from build123d import *

# Parameters (mm, degrees)
EXTRUDE_1_DEPTH = 3


with BuildPart() as part:
    # 草图1 → 凸台-拉伸1 (new body)
    with BuildSketch(Plane.XY):
        Polygon((120, -3), (80, -3), (80, 0), (61.5, 0), (61.5, -3), (62.75, -3), (62.75, -7), (61.5, -7), (61.5, -12), (58.5, -12), (58.5, -7), (57.25, -7), (57.25, -3), (58.5, -3), (58.5, 0), (40, 0), (40, -3), (0, -3), (0, -40), (3, -40), (3, -80), (0, -80), (0, -120), (3, -120), (3, -160), (0, -160), (0, -197), (40, -197), (40, -200), (58.5, -200), (58.5, -197), (57.25, -197), (57.25, -193), (58.5, -193), (58.5, -188), (61.5, -188), (61.5, -193), (62.75, -193), (62.75, -197), (61.5, -197), (61.5, -200), (80, -200), (80, -197), (120, -197), (120, -200), (138.5, -200), (138.5, -197), (137.25, -197), (137.25, -193), (138.5, -193), (138.5, -188), (141.5, -188), (141.5, -193), (142.75, -193), (142.75, -197), (141.5, -197), (141.5, -200), (160, -200), (160, -197), (200, -197), (200, -160), (197, -160), (197, -120), (200, -120), (200, -80), (197, -80), (197, -40), (200, -40), (200, -3), (160, -3), (160, 0), (141.5, 0), (141.5, -3), (142.75, -3), (142.75, -7), (141.5, -7), (141.5, -12), (138.5, -12), (138.5, -7), (137.25, -7), (137.25, -3), (138.5, -3), (138.5, 0), (120, 0), align=None)
    extrude(amount=EXTRUDE_1_DEPTH)


solid = part.part
The model under review builds one solid part; all positions refer to its coordinate system, in mm. Coordinates: 2 decimals unless noted, no trailing zeros. Write each loop counter-clockwise with the first axis right and the second up, starting at its lowest first coordinate (ties: lowest second). Pieces come first, ordered by that corner, then holes. Notation, with made-up numbers: (-6, 0.25) - (30, 0.25) arc R9 ccw to (30, 6.25) - close; hole circle Ø5 at (4, 87). An arc over 180 degrees is marked (long way). Answer as CSV lines item,"result".
(1) Clearance check with flat-ended pins moving along their axes: pin 1 Ø1.5 at (x, z) = (170, 2) entering from +Y; pin 2 Ø0.9 at (y, z) = (-148, 1.5) entering from -X; pin 3 Ø1.5 at (y, z) = (-198, 1) entering from +X. State where each tip first meets the part, or that it passes through.
Data:
pin 1,"stops at y = -3"
pin 2,"stops at x = 3"
pin 3,"stops at x = 160"
(2) We need section A-A (y = -126.5). Give the boundary of the cut face in (x, z), plus the area to 3 significant figures.
Data:
outline,"(3, 0) - (197, 0) - (197, 3) - (3, 3) - close"
area,"582 mm2"
(3) We need section B-B (x = 177.5). Give the boundary of the cut face in (y, z).
Data:
outline,"(-197, 0) - (-3, 0) - (-3, 3) - (-197, 3) - close"
(4) For line 1 along Y through (x, z) = (138, 0.9); line 2 along Y through (x, z) = (83, 0.4); line 3 along X through (y, z) = (-41, 2.5), list the stretches that pass through material, from the lowest coordinate up. Write a range as [from, to].
Data:
line 1,"y = [-200, -197], [-193, -7], [-3, 0]"
line 2,"y = [-197, -3]"
line 3,"x = [3, 197]"
